Here's how the part is built. I have some questions about the finished solid (model axes, mm). A direction names the side the tool comes from. Give positions to 0.01 mm unless a question says otherwise; leave off trailing zeros. Answer as CSV lines item,"result". Start each with the question number.
Q1. If I drill on line 1 along Y through (x, z) = (54, -1); line 2 along Y through (x, z) = (-53, -13); line 3 along Z through (x, y) = (-131, 90), over which ranges is the centre line in solid material (lowest first)?
Q2. For pin 1 (12 mm diameter, centred on x = -141, z = -18.5, fed in from -Y); pin 2 (8.5 mm diameter, centred on x = 110, y = 3, fed in from -Z); pin 3 (1.5 mm diameter, centred on x = -92.5, y = 0.5, fed in from -Z), each with a flat end and sliding along its axis, tell me the tip position at first contact or that it passes through.
Q3. Suppose I cut it at A-A (y = 0). Count the separate pieces of the cut face and the enclosed holes in it, then the cut area to 3 significant figures.
Q4. Thinking about a two-plate mould opening in X: for faces 1 (the cylindrical face through (39.96, -1.76, -34.18)), 2 (the cylindrical face through (-58.36, 90.18, -3.45)), 3 (the flat face through (-18, -88, 0)), 4 (the flat face through (48, -93, -7)), which applies, +X half, -X half, draft (parallel to the pull), parting line (faces both ways), or undercut?
Q5. On a 3-axis mill with a long thin cutter (end or side, diameter ignored), from which of +Z, -Z, +X, -X, +Y, -Y can I reach the whole of each face in a straight line? I mean faces 5 (the flat face through (-37, -1, -8)), 6 (the cylindrical face through (4.036, -30.736, -38.126)), 7 (the cylindrical face through (-113.495, 0.242, -3.451)). Say none if no direction works.
```python
from build123d import *

# Parameters (mm, degrees)
SKETCH_3_R                = 77
SKETCH_3_R_2              = 70
CUT_EXTRUDE_1_DEPTH       = 4
HOLE_WIZARD_1_D           = 11
HOLE_WIZARD_1_CBORE_D     = 17
HOLE_WIZARD_1_CBORE_DEPTH = 11
FILLET_1_R                = 2
CHAMFER_1_SIZE            = 2


with BuildPart() as part:
    # 草图1 → 旋转1 (revolve)
    with BuildSketch(Plane(origin=(0, 0, 0), x_dir=(0, 0, -1), z_dir=(1, 0, 0)), mode=Mode.PRIVATE) as revolve_1_sk:
        Polygon((0, 0), (0, 118), (8, 118), (8, 160), (11.526539614, 180), (18, 180), (18, 45), (21, 45), (21, 40), (47, 40), (47, 0), align=None)
    revolve(revolve_1_sk.sketch.rotate(Axis((0, 0, -47), (0, 0, 1)), 90), axis=Axis((0, 0, -47), (0, 0, 1)))

    # 草图2 → 切除-旋转1 (revolve, cut)
    with BuildSketch(Plane(origin=(0, 0, 0), x_dir=(0, 0, -1), z_dir=(1, 0, 0)), mode=Mode.PRIVATE) as cut_revolve_1_sk:
        Polygon((0, 0), (0, 88), (8, 88), (8, 28), (29, 28), (29, 31), (47, 31), (47, 0), align=None)
    revolve(cut_revolve_1_sk.sketch.rotate(Axis((0, 0, -47), (0, 0, 1)), 90), axis=Axis((0, 0, -47), (0, 0, 1)), mode=Mode.SUBTRACT)

    # 草图3 → 切除-拉伸1 (cut)
    with BuildSketch(Plane(origin=(0, 0, -18), x_dir=(-1, 0, 0), z_dir=(0, 0, -1))):
        Circle(SKETCH_3_R)
        Circle(SKETCH_3_R_2, mode=Mode.SUBTRACT)
    extrude(amount=-CUT_EXTRUDE_1_DEPTH, mode=Mode.SUBTRACT)

    # 孔1 (through all)
    with Locations(Plane(origin=(0, 0, -18), x_dir=(-1, 0, 0), z_dir=(0, 0, -1))):
        with Locations((54, 93.530743609), (108, 0), (54, -93.530743609), (-54, -93.530743609), (-108, 0), (-54, 93.530743609)):
            CounterBoreHole(HOLE_WIZARD_1_D / 2, HOLE_WIZARD_1_CBORE_D / 2, HOLE_WIZARD_1_CBORE_DEPTH)

    # 圆角1
    fillet_1_edges = [part.edges().sort_by_distance(p)[0] for p in [
        (88, 0, -8),
    ]]
    fillet(fillet_1_edges, radius=FILLET_1_R)

    # 倒角1
    chamfer_1_edges = [part.edges().sort_by_distance(p)[0] for p in [
        (28, 0, -8),
    ]]
    chamfer(chamfer_1_edges, length=CHAMFER_1_SIZE)


solid = part.part
```
Resolved:
1,line 1,"-104.92 to -99.03, -88.03 to -69.48, 69.48 to 88.03, 99.03 to 104.92"
1,line 2,"-172.02 to -101.97, -85.09 to 85.09, 101.97 to 172.02"
1,line 3,"-18 to -8"
2,pin 1,"y = -119.04"
2,pin 2,"z = -7"
2,pin 3,"z = -18"
3,separate pieces,"4"
3,enclosed holes,"0"
3,area,"3,480 mm^2"
4,face 1,"parting line"
4,face 2,"undercut"
4,face 3,"draft"
4,face 4,"undercut"
5,face 5,"+Z"
5,face 6,"-Z"
5,face 7,"+Z, -Z"
